Input: part model. Units: mm. Frame: model coordinates. Face numbers are marked on the shaded views. Round coordinates to 2 decimals unless told otherwise and drop trailing zeros. Loops run counter-clockwise (first coordinate to the right, second up) from the corner with the lowest first, then second, coordinate; pieces in that order, holes last. Notation, with made-up numbers: (-39.75, 43.5) -> (-20.75, 43.5) arc R37 cw to (-20.75, 80.5) -> close; hole circle Ø1 at (17.5, 60). An arc over 180 degrees is marked (long way). Answer in a Markdown table with one row per item. Add a question column.
Q1. Mould query, pull axis X, two halves, no side actions, for the marked faces 1, 2, 3 and 4. Classes: pulls with the +X half, pulls with the -X half, needs draft (parallel to the pull), parting line crosses it, or undercut.
Q2. Ray query, L1, parallel to Z at x = 0, y = -10.75; L2, parallel to Y at x = -0.5, z = -1; L3, parallel to Z at x = -1, y = -10.5. Return the intervals inside material, ascending. Write a range as from..to.
Q3. Pin query (flat end, axial travel): pin 1 (1 mm diameter, centred on y = 1.5, z = 0, fed in from -X); pin 2 (2 mm diameter, centred on x = -3, z = -3, fed in from +Y); pin 3 (1 mm diameter, centred on y = 2, z = 0, fed in from +X). Return the tip coordinate at first contact, or that it passes through.
Q4. Section A-A, the plane y = -7.5. Output: boundary loops of the cut face in (x, z), and give its area (3 significant figures).
```python
from build123d import *

# Parameters (mm, degrees)
CUT_EXTRUDE1_DEPTH = 1.27


with BuildPart() as part:
    # Sketch1 → Revolve1 (revolve)
    with BuildSketch(Plane.XY):
        with BuildLine():
            Line((-2.0828, 0), (-3.9624, 0))
            ThreePointArc((-3.9624, 0), (-3.131232795, 1.352726455), (-1.79477003, 2.2098))
            Line((-1.79477003, 2.2098), (0, 2.2098))
            Line((0, 2.2098), (0, -19.05))
            Line((0, -19.05), (-2.0828, -19.05))
            Line((-2.0828, -19.05), (-2.0828, 0))
        make_face()
    revolve(axis=Axis((0, -19.05, 0), (0, 1, 0)))

    # Sketch2 → Cut-Extrude1 (cut)
    with BuildSketch(Plane(origin=(0, 2.2098, 0), x_dir=(1, 0, 0), z_dir=(0, 1, 0))):
        Polygon((-1.190625, 0.687407664), (-1.190625, -0.687407664), (0, -1.374815329), (1.190625, -0.687407664), (1.190625, 0.687407664), (0, 1.374815329), align=None)
    extrude(amount=-CUT_EXTRUDE1_DEPTH, mode=Mode.SUBTRACT)


solid = part.part
```
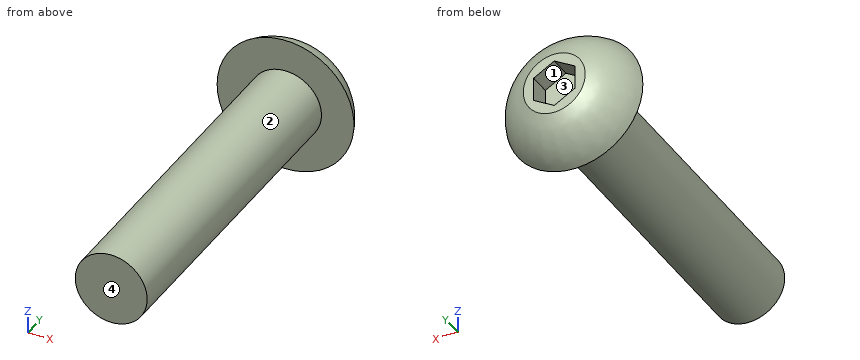
Answer block:
| question | item | result |
|---|---|---|
| 1 | face 1 | undercut |
| 1 | face 2 | parting line crosses it |
| 1 | face 3 | undercut |
| 1 | face 4 | needs draft |
| 2 | L1 | -2.08..2.08 |
| 2 | L2 | -19.05..0.94 |
| 2 | L3 | -1.83..1.83 |
| 3 | pin 1 | x = -3.43 |
| 3 | pin 2 | y = 1.23 |
| 3 | pin 3 | x = 2.98 |
| 4 | outline | circle Ø4.17 at (0, 0) |
| 4 | area | 13.6 mm^2 |
